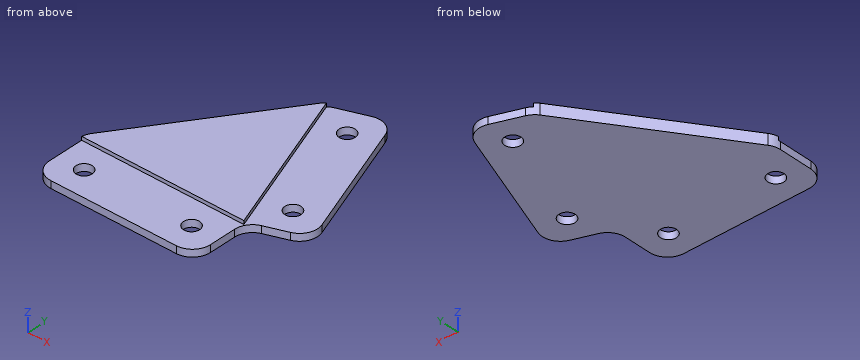
from build123d import *

# Parameters (mm, degrees)
EXTRUDE_1_DEPTH     = 3
SKETCH_2_R          = 2.25
CUT_EXTRUDE_1_DEPTH = 3
FILLET_1_R          = 5
CUT_EXTRUDE_2_DEPTH = 1


with BuildPart() as part:
    # ｽｹｯﾁ1 → ﾎﾞｽ - 押し出し1 (new body)
    with BuildSketch(Plane.XY):
        Polygon((440, 0), (440, -16), (395, -16), (395, 0), (424.60909355, 42.286167935), (438.704482862, 47.416470085), (454.095389312, 5.13030215), align=None)
    extrude(amount=EXTRUDE_1_DEPTH)

    # ｽｹｯﾁ2 → ｶｯﾄ - 押し出し1 (cut)
    with BuildSketch(Plane.XY.offset(3)):
        with Locations((402.5, -8.5)):
            Circle(SKETCH_2_R)
        with Locations((432.5, -8.5)):
            Circle(SKETCH_2_R)
        with Locations((434.221939281, 37.803624354)):
            Circle(SKETCH_2_R)
        with Locations((444.482543581, 9.612845731)):
            Circle(SKETCH_2_R)
    extrude(amount=-CUT_EXTRUDE_1_DEPTH, mode=Mode.SUBTRACT)

    # ﾌｨﾚｯﾄ1
    fillet_1_edges = [part.edges().sort_by_distance(p)[0] for p in [
        (395, -16, 1.5),
        (395, 0, 1.5),
        (424.60909355, 42.286167935, 1.5),
        (438.704482862, 47.416470085, 1.5),
        (454.095389312, 5.13030215, 1.5),
        (440, 0, 1.5),
        (440, -16, 1.5),
    ]]
    fillet(fillet_1_edges, radius=FILLET_1_R)

    # ｽｹｯﾁ4 → ｶｯﾄ - 押し出し2 (cut)
    with BuildSketch(Plane.XY.offset(3)):
        Polygon((438.704482862, 47.416470085), (455.121449742, 2.311224288), (443, -2.100622615), (443, -16), (395, -16), (395, -0.95), (440.292562834, -0.95), (424.562108919, 42.269066928), align=None)
    extrude(amount=-CUT_EXTRUDE_2_DEPTH, mode=Mode.SUBTRACT)


solid = part.part
Geometry: final body of the model. Coordinates: model frame, mm. Give positions to 0.01 mm unless a question says otherwise; leave off trailing zeros. Write each loop counter-clockwise with the first axis right and the second up, starting at its lowest first coordinate (ties: lowest second). Pieces come first, ordered by that corner, then holes.
(1) First-contact query: P1, Ø1, axis at y = 32.5, z = 2.5, coming from the -X side; P2, Ø0.6, axis at y = -6.5, z = 1, coming from the +X side; P3, Ø12, axis at x = 437, y = -7, coming from the +Z side; P4, Ø2.5, axis at x = 444.48, y = 9.61, coming from the +Z side. Flat tips, straight axial feed; report the tip coordinate or a pass-through.
(2) Cut plane D-D, the plane x = 416.5. Return loops of the section in (y, z), then the cut area to 3 significant figures.
(3) Cut plane C-C, the plane z = 0.65. Return loops of the section in (x, y), then the cut area to 3 significant figures.
(4) Cut plane A-A, the plane y = -8.5. Return loops of the section in (x, z).
(5) Ray query, line 1 (Y direction, x = 432.5, z = 1.15); line 2 (Z direction, x = 441.5, y = 27); line 3 (X direction, y = 36, z = 0.75). Return the intervals inside material, ascending.
(6) Cut plane B-B, the plane x = 446. Return loops of the section in (y, z).
Values follow:
1. P1: stops at x = 417.41
1. P2: stops at x = 440
1. P3: stops at z = 2
1. P4: passes through
2. outline: (-16, 0) - (30.71, 0) - (30.71, 3) - (-0.95, 3) - (-0.95, 2) - (-16, 2) - close
2. area: 125 mm2
3. outline: (395, -11) arc R5 ccw to (400, -16) - (435, -16) arc R5 ccw to (440, -11) - (440, -3.5) arc R5 cw to (443.29, 1.2) - (449.4, 3.42) arc R5 ccw to (452.39, 9.83) - (440.41, 42.72) arc R5 ccw to (434.01, 45.71) - (426.09, 42.83) arc R5 ccw to (423.7, 40.99) - (395.9, 1.29) arc R5 ccw to (395, -1.58) - close; hole circle Ø4.5 at (402.5, -8.5); hole circle Ø4.5 at (432.5, -8.5); hole circle Ø4.5 at (434.22, 37.8); hole circle Ø4.5 at (444.48, 9.61)
3. area: 2,260 mm2
4. outline: (395, 0) - (400.25, 0) - (400.25, 2) - (395, 2) - close; (404.75, 0) - (430.25, 0) - (430.25, 2) - (404.75, 2) - close; (434.75, 0) - (440, 0) - (440, 2) - (434.75, 2) - close
5. line 1: y = -16 to -10.75, -6.25 to 36.36, 39.25 to 45.16
5. line 2: z = 0 to 2
5. line 3: x = 420.21 to 432.88, 435.57 to 442.86
6. outline: (2.18, 0) - (7.95, 0) - (7.95, 2) - (2.18, 2) - close; (11.27, 0) - (27.37, 0) - (27.37, 2) - (11.27, 2) - close
